Build history of the part. All positions in model axes, mm. Round coordinates to 2 decimals unless told otherwise and drop trailing zeros. Loops run counter-clockwise (first coordinate to the right, second up) from the corner with the lowest first, then second, coordinate; pieces in that order, holes last. Notation, with made-up numbers: M 82,-28.75 L 106,-28.75 A31 ccw 106,3.25 Z; hole C -38.5,44.25 d6. An arc over 180 degrees is marked long. One line per item, written item: value.
```python
from build123d import *

# Parameters (mm, degrees)
SKICA2_W                = 0.5
SKICA2_H                = 0.5
P_IDAT_VYSUNUT_M1_DEPTH = 1.9


with BuildPart() as part:
    # Skica1 → Rotovat1 (revolve)
    with BuildSketch(Plane.XY, mode=Mode.PRIVATE) as rotovat1_sk:
        with BuildLine():
            Line((0, 0), (0, 2.75))
            ThreePointArc((0, 2.75), (0.146446609, 3.103553391), (0.5, 3.25))
            Line((0.5, 3.25), (0.749493844, 3.25))
            ThreePointArc((0.749493844, 3.25), (1.063131818, 3.233560159), (1.373332352, 3.184420814))
            add(Edge.make_bspline(
                [(1.373332352, 3.184420814), (1.844148672, 3.08432837), (2.637509596, 2.913100219), (3.679859415, 3.18917118), (4.202566014, 3.237341565)],
                knots=[0.049740357, 0.049740357, 0.049740357, 0.049740357, 0.292962234, 0.585924467, 0.585924467, 0.585924467, 0.585924467], degree=3))
            ThreePointArc((4.202566014, 3.237341565), (4.340070837, 3.24683372), (4.477866527, 3.25))
            Line((4.477866527, 3.25), (6.9, 3.25))
            ThreePointArc((6.9, 3.25), (7.253553391, 3.103553391), (7.4, 2.75))
            Line((7.4, 2.75), (7.4, 0))
            Line((7.4, 0), (0, 0))
        make_face()
    revolve(rotovat1_sk.sketch.rotate(Axis((7.4, 0, 0), (-1, 0, 0)), 90), axis=Axis((7.4, 0, 0), (-1, 0, 0)))

    # Skica2 → Přidat vysunutím1 (add)
    with BuildSketch(Plane.ZY):
        with Locations((0, -1.2)):
            Rectangle(SKICA2_W, SKICA2_H)
        with Locations((0, 1.2)):
            Rectangle(SKICA2_W, SKICA2_H)
    extrude(amount=P_IDAT_VYSUNUT_M1_DEPTH)


solid = part.part
```
Item 1: Slice it at A-A, the plane x = -0.5. Give the cut face in (y, z), and give its area (3 significant figures).
Check values:
outline: M -1.45,-0.25 L -0.95,-0.25 L -0.95,0.25 L -1.45,0.25 Z; M 0.95,-0.25 L 1.45,-0.25 L 1.45,0.25 L 0.95,0.25 Z
area: 0.500 mm2
Item 2: Drop flat-ended pins along their axis: P1, Ø1.6, axis at y = -0.5, z = -1, coming from the -X side; P2, Ø2, axis at x = 2.5, y = 0, coming from the +Z side; P3, Ø0.6, axis at x = -1, z = 0, coming from the +Y side. Give the stop position or say it passes through.
Check values:
P1: stops at x = 0
P2: stops at z = 3.16
P3: stops at y = 1.45
Item 3: Slice it at B-B, the plane x = 5.25. Give the cut face in (y, z), and give its area (3 significant figures).
Check values:
outline: C 0,0 d6.5
area: 33.2 mm2
Item 4: Wall check: line 1 along X through (y, z) = (1.75, 0.75); line 2 along Z through (x, y) = (-0.5, -1); line 3 along Z through (x, y) = (5.5, -2.5). Give the ranges that are in metal, low to high.
Check values:
line 1: x = 0 to 7.4
line 2: z = -0.25 to 0.25
line 3: z = -2.08 to 2.08
